Input: part model. Units: mm. Frame: model coordinates. Face numbers are marked on the shaded views. A direction names the side the tool comes from. Give positions to 0.01 mm unless a question says otherwise; leave off trailing zeros. Loops run counter-clockwise (first coordinate to the right, second up) from the corner with the lowest first, then second, coordinate; pieces in that order, holes last. Notation, with made-up numbers: (19.5, 24) - (61.5, 24) arc R24 ccw to (61.5, 36) - close; hole circle Ø6 at (-3.75, 58). An arc over 180 degrees is marked (long way). Answer as a JSON object with one key per item and string values. Group by question number.
(1) Access query for the marked faces 4, 5, 6 and 7. Directions: +Z, -Z, +X, -X, +Y, -Y. A direction counts if a zero-diameter tool reaches every point of the face in a straight line with its end or side. Return the directions, or none.
(2) Section query B-B (y = 0). Return loops of the section in (x, z).
(3) Material intervals for L1, parallel to Z at x = -1.5, y = 4.5; L2, parallel to Y at x = -2, z = 17.75; L3, parallel to Y at x = -4.25, z = 11, sorted ascending.
(4) Mould query, pull axis X, two halves, no side actions, for the marked faces 1, 2 and 3. Classes: +X half, -X half, draft (parallel to the pull), parting line (faces both ways), or undercut.
(5) Section query A-A (z = 12.75). Return loops of the section in (x, y), plus the area to 3 significant figures.
(6) Pin query (flat end, axial travel): P1, Ø8, axis at y = 2.5, z = 16, coming from the -X side; P2, Ø3, axis at x = -3, z = 14.5, coming from the +Y side; P3, Ø6, axis at y = -0.5, z = 16, coming from the +X side. Return the tip coordinate at first contact, or that it passes through.
```python
from build123d import *

# Parameters (mm, degrees)
CROQUIS1_R              = 7
SALIENTE_EXTRUIR1_DEPTH = 5
CROQUIS2_R              = 4.75
SALIENTE_EXTRUIR2_DEPTH = 15
CHAFL_N1_SIZE           = 2
CHAFL_N1_SIZE2          = 2.22122503
CORTAR_EXTRUIR1_START   = -15
CORTAR_EXTRUIR1_DEPTH   = 15
MATRIZC1_COUNT          = 12


with BuildPart() as part:
    # Croquis1 → Saliente-Extruir1 (new body)
    with BuildSketch(Plane.XY):
        Circle(CROQUIS1_R)
    extrude(amount=SALIENTE_EXTRUIR1_DEPTH)

    # Croquis2 → Saliente-Extruir2 (add)
    with BuildSketch(Plane.XY.offset(5)):
        Circle(CROQUIS2_R)
    extrude(amount=SALIENTE_EXTRUIR2_DEPTH)

    # Chaflán1
    chafl_n1_edges = [part.edges().sort_by_distance(p)[0] for p in [
        (-7, 0, 5),
    ]]
    chafl_n1_side = [part.faces().sort_by_distance(p)[0] for p in [
        (-7, 0, 2.5),
    ]]
    chamfer(chafl_n1_edges, length=CHAFL_N1_SIZE, length2=CHAFL_N1_SIZE2, reference=chafl_n1_side[0])

    # Croquis3 → Cortar-Extruir1 (cut)
    with BuildSketch(Plane.XY.offset(20).offset(CORTAR_EXTRUIR1_START)):
        with BuildLine():
            ThreePointArc((-0.941424284, 4.655772795), (0.03975399, 4.467490129), (1.024127494, 4.638282319))
            ThreePointArc((1.024127494, 4.638282319), (0.042266233, 4.749811951), (-0.941424284, 4.655772795))
        make_face()
    cortar_extruir1 = extrude(amount=CORTAR_EXTRUIR1_DEPTH, mode=Mode.SUBTRACT)

    # MatrizC1: Cortar-Extruir1 ×12 about axis
    matrizc1_axis = Axis((0, 0, 0), (0, 0, 1))
    for i in range(1, MATRIZC1_COUNT):
        add(cortar_extruir1.rotate(matrizc1_axis, i * 360 / MATRIZC1_COUNT), mode=Mode.SUBTRACT)


solid = part.part
```
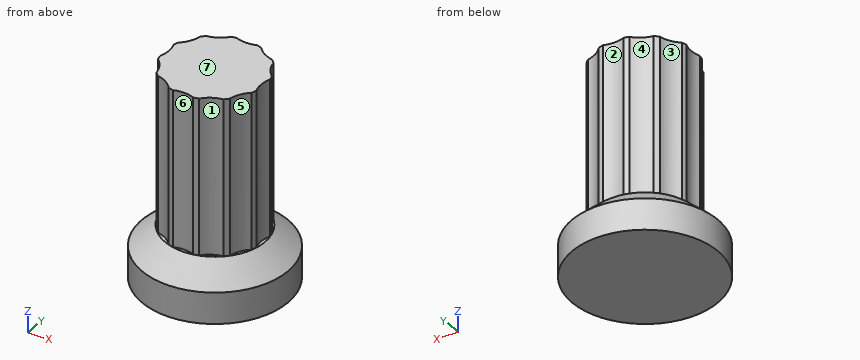
Recorded:
{
 "1": {"face 4": "+Z, -X, +Y", "face 5": "+Z, +X, -Y", "face 6": "+Z, -Y", "face 7": "+Z, +X, -X, +Y, -Y"},
 "2": {"outline": "(-7, 0) - (7, 0) - (7, 3) - (4.78, 5) - (4.47, 5) - (4.47, 20) - (-4.47, 20) - (-4.47, 5) - (-4.78, 5) - (-7, 3) - close"},
 "3": {"L1": "z = 0 to 5", "L2": "y = -4.03 to 4.01", "L3": "y = -1.7 to 1.74"},
 "4": {"face 1": "+X half", "face 2": "undercut", "face 3": "-X half"},
 "5": {"outline": "(-4.66, -0.94) arc R4.75 ccw to (-4.53, -1.43) arc R2.78 cw to (-3.56, -3.14) arc R4.75 ccw to (-3.21, -3.5) arc R2.78 cw to (-1.51, -4.5) arc R4.75 ccw to (-1.02, -4.64) arc R2.78 cw to (0.94, -4.66) arc R4.75 ccw to (1.43, -4.53) arc R2.78 cw to (3.14, -3.56) arc R4.75 ccw to (3.5, -3.21) arc R2.78 cw to (4.5, -1.51) arc R4.75 ccw to (4.64, -1.02) arc R2.78 cw to (4.66, 0.94) arc R4.75 ccw to (4.53, 1.43) arc R2.78 cw to (3.56, 3.14) arc R4.75 ccw to (3.21, 3.5) arc R2.78 cw to (1.51, 4.5) arc R4.75 ccw to (1.02, 4.64) arc R2.78 cw to (-0.94, 4.66) arc R4.75 ccw to (-1.43, 4.53) arc R2.78 cw to (-3.14, 3.56) arc R4.75 ccw to (-3.5, 3.21) arc R2.78 cw to (-4.5, 1.51) arc R4.75 ccw to (-4.64, 1.02) arc R2.78 cw to start", "area": "66.4 mm^2"},
 "6": {"P1": "stops at x = -4.66", "P2": "stops at y = 4.45", "P3": "stops at x = 4.66"}
}
